Verification items for the finished model (mm, model axes). A direction names the side the tool comes from. Round coordinates to 2 decimals unless told otherwise and drop trailing zeros. Write each loop counter-clockwise with the first axis right and the second up, starting at its lowest first coordinate (ties: lowest second). Pieces come first, ordered by that corner, then holes. Notation, with made-up numbers: (-28, -30) - (-4, -30) arc R23 ccw to (-4, 5) - close; hole circle Ø8 at (-24.5, -1.5). An arc over 180 degrees is marked (long way). Answer as a JSON object with one key per item and string values. Group by question number.
1) Set-up check for faces 1 (the flat face through (54.566, 17, 13)), 2 (the cylindrical face through (10.727, 20.823, 30.534)): record each of +Z, -Z, +X, -X, +Y, -Y from which the full face is reachable in a straight line by a thin tool's end or side.
2) Section check B-B (y = 30). Enter the section's corners in (x, z), then the cut area to 3 significant figures.
3) Section check C-C (z = 32.5). Enter the section's corners in (x, y).
4) Section check A-A (x = 12). Enter the section's corners in (y, z), then the cut area to 3 significant figures.
5) Section check D-D (y = 10). Enter the section's corners in (x, z), then the cut area to 3 significant figures.
6) Go/stop test with a flat-tipped pin: pin 1 Ø17 at (x, y) = (25, 15) entering from +Z. Record where the tip stops, or that it passes through.
7) Thickness scan on line 1 (Z direction, x = 52, y = 2.5); line 2 (X direction, y = 21, z = 27.5); line 3 (X direction, y = 27.5, z = 31.5). Record the ranges inside material, lowest first.
```python
from build123d import *

# Parameters (mm, degrees)
F0_W     = 54.566301
F0_H     = 33.538647
F1_DEPTH = 25.4
F2_R     = 6.13249
F3_DEPTH = 35.814


with BuildPart() as f1:
    # F0 (on Top) → F1 (new body)
    with BuildSketch(Plane.XY):
        with Locations((27.28315, 16.769323)):
            Rectangle(F0_W, F0_H)
    extrude(amount=F1_DEPTH)

    # F2 (on Top) → F3 (join)
    with BuildSketch(Plane.XY):
        with Locations((7.89733, 26.263695)):
            Circle(F2_R)
    extrude(amount=F3_DEPTH)


solid = f1.part
```
Returned:
{
 "1": {"face 1": "+Z, -Z, +X, +Y, -Y", "face 2": "+Z"},
 "2": {"outline": "(0, 0) - (54.57, 0) - (54.57, 25.4) - (12.76, 25.4) - (12.76, 35.81) - (3.03, 35.81) - (3.03, 25.4) - (0, 25.4) - close", "area": "1,490 mm2"},
 "3": {"outline": "circle Ø12.26 at (7.9, 26.26)"},
 "4": {"outline": "(0, 0) - (33.54, 0) - (33.54, 25.4) - (30.82, 25.4) - (30.82, 35.81) - (21.71, 35.81) - (21.71, 25.4) - (0, 25.4) - close", "area": "947 mm2"},
 "5": {"outline": "(0, 0) - (54.57, 0) - (54.57, 25.4) - (0, 25.4) - close", "area": "1,390 mm2"},
 "6": {"pin 1": "z = 25.4"},
 "7": {"line 1": "0 to 25.4", "line 2": "4.75 to 11.04", "line 3": "1.89 to 13.9"}
}
